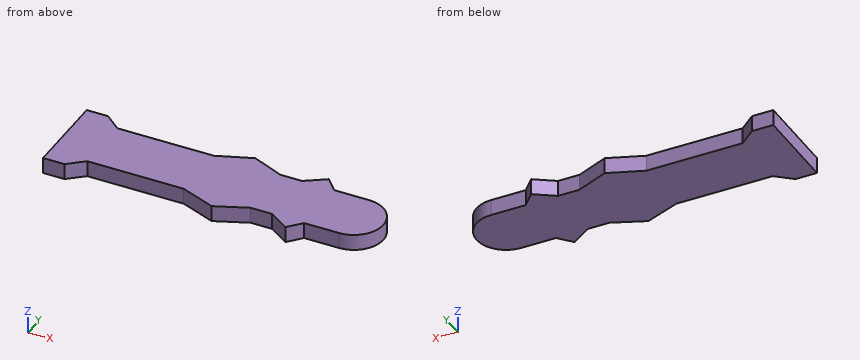
Autodesk Fusion 360 part; units mm, degrees
sketch "Sketch1" plane through (0, 0, 0) normal (0, 0, 1) x (1, 0, 0)
  line L0 (0, 0) -> (-119, 0)
  line L1 (-119, 0) -> (-119, 32)
  line L2 (-119, 32) -> (0, 32)
  line L3 (0, 32) -> (0, 0)
  line L4 (-105, 27.0131) -> (-111, 32)
  line L5 (-105, 27.0131) -> (-69, 27.0131)
  line L6 (-69, 27.0131) -> (-56, 32)
  line L7 (-105, 4.9869) -> (-69, 4.9869)
  line L8 (-105, 4.9869) -> (-111, 0)
  line L9 (-69, 4.9869) -> (-56, 0)
  line L10 (-44, 27) -> (-36, 27)
  line L11 (-44, 27) -> (-56, 32)
  line L12 (-36, 27) -> (-28.5, 32)
  line L13 (-28.5, 32) -> (-24, 27)
  line L14 (-24, 27) -> (0, 27)
  line L15 (-24, 5) -> (0, 5)
  line L16 (-28.5, 0) -> (-24, 5)
  line L17 (-36, 5) -> (-28.5, 0)
  line L18 (-44, 5) -> (-36, 5)
  line L19 (-44, 5) -> (-56, 0)
  circle A0 centre (-11, 16) radius 11
  dimension "d1" = 119
  dimension "d2" = 32
  dimension "d5" = 8
  dimension "d14" = 14
  dimension "d16" = 36
  dimension "d17" = 63
  dimension "d18" = 8
  dimension "d19" = 25
  dimension "d21" = 12
extrude "Extrude1" add sketch "Sketch1" along normal blind 6 contours L0 L1 L2 L4 L5 L6 L7 L8 L9 L10 L11 L12 L13 L14 L15 L16 L17 L18 L19 A0 | A0
equation "d16 = 50 mm - 14 mm"
The listing builds one solid part. Answer for the finished solid, in the listing's coordinates (mm). Coordinates: 2 decimals unless noted, no trailing zeros. Order: outer loops, then holes, each group sorted by start corner. A loop starts at its lowest first (then second) coordinate and runs counter-clockwise, first axis right, second up. Notation, with made-up numbers: M 34.25,11.25 L 59.25,11.25 A19 cw 59.25,41.25 Z; hole C 51,43.25 d3. An arc over 180 degrees is marked long. Answer as a JSON object with one key per item and string values. Group by question number.
1. Straight lines are drawn through the part: line 1 (Y direction, x = -82.5, z = 3.7); line 2 (X direction, y = 8, z = 4.35); line 3 (Y direction, x = -65, z = 1.6). For each, find the intervals that lie inside material, in ascending order.
2. Section B-B on y = 6.5 is taken. Write down the section's boundary in (x, z).
3. Section A-A on x = -17 is taken. Write down the section's boundary in (y, z), then the cut area to 3 significant figures.
4. Flat-ended cylindrical pins translate along their axes: P1, Ø3, axis at x = -41.5, z = 2.5, coming from the +Y side; P2, Ø1, axis at x = -51.5, z = 3, coming from the -Y side. Find the tip coordinate at first contact, or state that the pin passes through.
Values follow:
{
 "1": {"line 1": "4.99 to 27.01", "line 2": "-119 to -3.45", "line 3": "3.45 to 28.55"},
 "2": {"outline": "M -119,0 L -5.45,0 L -5.45,6 L -119,6 Z"},
 "3": {"outline": "M 5,0 L 27,0 L 27,6 L 5,6 Z", "area": "132 mm2"},
 "4": {"P1": "y = 27", "P2": "y = 1.67"}
}
